Source: CAD feature listing. Evaluate the final solid. Frame: model axes, mm. A direction names the side the tool comes from. Round coordinates to 2 decimals unless told otherwise and drop trailing zeros. Write each loop counter-clockwise with the first axis right and the second up, starting at its lowest first coordinate (ties: lowest second). Pieces come first, ordered by that corner, then holes. Notation, with made-up numbers: M 50.5,87 L 56.5,87 A18 cw 56.5,94 Z; hole C 10,9 d6. An arc over 180 degrees is marked long. Answer in a Markdown table with one row per item.
from build123d import *

# Parameters (mm, degrees)
SKETCH1_W                = 40
SKETCH1_H                = 20
BOSS_EXTRUDE1_DEPTH      = 40.5
BOSS_EXTRUDE2_DEPTH      = 5.75
BOSS_EXTRUDE2_DEPTH_BACK = 46.25
SKETCH2_R                = 2.5
BOSS_EXTRUDE3_DEPTH      = 2
BOSS_EXTRUDE3_DEPTH_BACK = 42.5
SKETCH3_R                = 1


with BuildPart() as part:
    # Sketch1 → Boss-Extrude1 (new body)
    with BuildSketch(Plane(origin=(0, 0, 0), x_dir=(1, 0, 0), z_dir=(0, 1, 0))):
        with Locations((3.756737992, 0.753901676)):
            Rectangle(SKETCH1_W, SKETCH1_H)
    extrude(amount=BOSS_EXTRUDE1_DEPTH)

    # Sketch2 → Boss-Extrude2 (add, two sides: drawn at the far end of the back side and taken through both)
    with BuildSketch(Plane(origin=(0, 40.5, 0), x_dir=(1, 0, 0), z_dir=(0, 1, 0)).offset(-BOSS_EXTRUDE2_DEPTH_BACK)):
        with Locations(Location((13.756737992, 0.753901676, 0), (0, 0, 270))):
            Circle(SKETCH2_R)
    extrude(amount=BOSS_EXTRUDE2_DEPTH + BOSS_EXTRUDE2_DEPTH_BACK)

    # Sketch3 → Boss-Extrude3 (add, two sides: drawn at the far end of the back side and taken through both)
    with BuildSketch(Plane(origin=(0, 40.5, 0), x_dir=(1, 0, 0), z_dir=(0, 1, 0)).offset(-BOSS_EXTRUDE3_DEPTH_BACK)):
        with Locations(Location((-13.243262008, 1.180776093, 0), (0, 0, 270))):
            Circle(SKETCH3_R)
        with Locations(Location((-6.243262008, 7.753901676, 0), (0, 0, 270))):
            Circle(SKETCH3_R)
        with Locations(Location((-6.243262008, -6.246098324, 0), (0, 0, 270))):
            Circle(SKETCH3_R)
    extrude(amount=BOSS_EXTRUDE3_DEPTH + BOSS_EXTRUDE3_DEPTH_BACK)


solid = part.part
Q1. Section C-C (x = 14.5). Return loops of the section in (y, z), and give its area (3 significant figures).
Solutions:
| item | result |
|---|---|
| outline | M -5.75,-3.14 L 0,-3.14 L 0,-10.75 L 40.5,-10.75 L 40.5,-3.14 L 46.25,-3.14 L 46.25,1.63 L 40.5,1.63 L 40.5,9.25 L 0,9.25 L 0,1.63 L -5.75,1.63 Z |
| area | 865 mm2 |
Q2. Contact query for flat-ended pins moving along their axis: pin 1 Ø1 at (x, z) = (-6.5, -8) entering from -Y; pin 2 Ø2 at (x, z) = (-13, -1.5) entering from +Y; pin 3 Ø1 at (x, z) = (-0.5, 4) entering from -Y. Output: stop coordinate, or through.
Solutions:
| item | result |
|---|---|
| pin 1 | stops at y = -2 |
| pin 2 | stops at y = 42.5 |
| pin 3 | stops at y = 0 |
Q3. Section A-A (z = 1). Return loops of the section in (x, y), and give its area (3 significant figures).
Solutions:
| item | result |
|---|---|
| outline | M -16.24,0 L 11.98,0 L 11.98,-5.75 L 15.54,-5.75 L 15.54,0 L 23.76,0 L 23.76,40.5 L 15.54,40.5 L 15.54,46.25 L 11.98,46.25 L 11.98,40.5 L -16.24,40.5 Z |
| area | 1,660 mm2 |
Q4. Material intervals for probe 1 along Y at (x, z) = (12, 6.25); probe 2 along Y at (x, z) = (-12.5, -1.25); probe 3 along Z at (x, y) = (13, -1), sorted ascending.
Solutions:
| item | result |
|---|---|
| probe 1 | y = 0 to 40.5 |
| probe 2 | y = -2 to 42.5 |
| probe 3 | z = -3.14 to 1.63 |
Q5. Pull-direction query (Z, two-part tool) for faces 5 (the flat face through (3, 20, -10.754)), 6 (the cylindrical face through (-5.567, -1.014, 5.509)), 7 (the flat face through (23.757, 20, -1)), 8 (the cylindrical face through (11.316, 43.335, -1.296)); classes: pulls with the +Z half, pulls with the -Z half, needs draft (parallel to the pull), parting line crosses it, or undercut.
Solutions:
| item | result |
|---|---|
| face 5 | pulls with the -Z half |
| face 6 | undercut |
| face 7 | needs draft |
| face 8 | parting line crosses it |
Q6. Section D-D (x = 6.5). Return loops of the section in (y, z).
Solutions:
| item | result |
|---|---|
| outline | M 0,-10.75 L 40.5,-10.75 L 40.5,9.25 L 0,9.25 Z |
Q7. Access query for faces 1 (the flat face through (-13, 42.5, -1)), 2 (the cylindrical face through (11.316, -2.915, -1.296)), 3 (the flat face through (-13, -2, -1)), 4 (the cylindrical face through (-5.567, 41.486, 5.509)). Directions: +Z, -Z, +X, -X, +Y, -Y. A direction counts if a zero-diameter tool reaches every point of the face in a straight line with its end or side. Return the directions, or none.
Solutions:
| item | result |
|---|---|
| face 1 | +Z, -Z, -X, +Y |
| face 2 | -Y |
| face 3 | +Z, -Z, -X, -Y |
| face 4 | +Y |
Q8. Section B-B (y = -1). Return loops of the section in (x, z), and give its area (3 significant figures).
Solutions:
| item | result |
|---|---|
| outline | C -13.24,-1.18 d2; C -6.24,-7.75 d2; C -6.24,6.25 d2; C 13.76,-0.75 d5 |
| area | 29.1 mm2 |
